Work out the finished part from the listing and answer in its coordinate system (mm). A direction names the side the tool comes from. Round coordinates to 2 decimals unless told otherwise and drop trailing zeros. Order: outer loops, then holes, each group sorted by start corner. A loop starts at its lowest first (then second) coordinate and runs counter-clockwise, first axis right, second up. Notation, with made-up numbers: (41.5, -18.5) - (86.5, -18.5) arc R3 cw to (86.5, -14.5) - close; hole circle Ø7 at (2, 88). An arc over 180 degrees is marked (long way). Use CSV: the item, a comma, the result in double quotes.
from build123d import *

# Parameters (mm, degrees)
F1_DEPTH = 80
F2_SIZE  = 60
F3_R     = 10
F4_R     = 10
F5_DEPTH = 25


with BuildPart() as f1:
    # F0 (on Right) → F1 (new body)
    with BuildSketch(Plane.YZ):
        Polygon((4191.274234, 1023.006535), (1401.929079, 1267.042615), (1391.47039, 1147.499251), (1789.291577, 1112.694407), (1889.291577, 1112.694407), (1889.291577, 1103.945541), (3689.291577, 946.465946), (3789.291577, 946.465946), (3789.291577, 937.71708), (4180.815545, 903.463171), align=None)
    extrude(amount=F1_DEPTH)

    # F2
    f2_edges = [f1.edges().sort_by_distance(p)[0] for p in [
        (40, 1391.47039, 1147.499251),
        (40, 4180.815545, 903.463171),
    ]]
    chamfer(f2_edges, length=F2_SIZE)

    # F3 (on face) + F4 (on face) → F5 (cut)
    with BuildSketch(Plane(origin=(0, 0, 1112.694407), x_dir=(1, 0, 0), z_dir=(0, 0, -1))):
        with Locations((40, -1839.291577)):
            Circle(F3_R)
    with BuildSketch(Plane(origin=(0, 0, 946.465946), x_dir=(1, 0, 0), z_dir=(0, 0, -1))):
        with Locations((40, -3739.291577)):
            Circle(F4_R)
    extrude(amount=-F5_DEPTH, mode=Mode.SUBTRACT)


solid = f1.part
(1) For faces 1 (the flat face through (39, 1827, 1112.694)), 2 (the flat face through (80, 2787, 1089)), determine the directions among +Z, -Z, +X, -X, +Y, -Y from which every point of the face is accessible in a straight line to the end or side of a thin tool.
Findings below:
face 1,"-Z, +X, -X, -Y"
face 2,"+Z, -Z, +X, +Y, -Y"
(2) Find section A-A (z = 1232.5). Determine the outline of the cut face in (x, y), and give its area (3 significant figures).
Findings below:
outline,"(0, 1398.91) - (80, 1398.91) - (80, 1796.75) - (0, 1796.75) - close"
area,"31,800 mm²"
(3) Find section B-B (y = 1675.5). Determine the outline of the cut face in (x, z), and give its area (3 significant figures).
Findings below:
outline,"(0, 1122.65) - (80, 1122.65) - (80, 1243.11) - (0, 1243.11) - close"
area,"9,640 mm²"
(4) Find the intervals of material crossed by L1, parallel to Z at x = 61.5, y = 3727.5; L2, parallel to Z at x = 45.5, y = 1819.5, in increasing order. Write a range as from..to.
Findings below:
L1,"z = 946.47..1063.58"
L2,"z = 1112.69..1230.51"
(5) Each of these flat-tipped pins is pushed along its axis until it touches: pin 1 (6 mm diameter, centred on x = 29.5, z = 1215, fed in from -Y); pin 2 (16 mm diameter, centred on x = 40, y = 1839.29, fed in from -Z); pin 3 (4.5 mm diameter, centred on x = 37.5, z = 943, fed in from -Y). Where does it stop, or does it pass through?
Findings below:
pin 1,"stops at y = 1397.11"
pin 2,"stops at z = 1137.69"
pin 3,"stops at y = 3789.29"
